Source: three-view drawing plus pictorial views. Frame: mm from the lowest corner of the part. A direction names the side the tool comes from. Round coordinates to 2 decimals unless told otherwise and drop trailing zeros. Loops run counter-clockwise (first coordinate to the right, second up) from the corner with the lowest first, then second, coordinate; pieces in that order, holes last. Notation, with made-up numbers: (65.5, 66.25) -> (84.5, 66.25) arc R27 ccw to (84.5, 100.25) -> close; hole circle Ø1 at (77, 34.5). An arc over 180 degrees is marked (long way). Put each result on its own line as item: value. Start each with the question number.
1. Contact query for flat-ended pins moving along their axis: pin 1 (2 mm diameter, centred on y = 2, z = 35.5, fed in from +X); pin 2 (2 mm diameter, centred on y = 7, z = 34.5, fed in from +X); pin 3 (2 mm diameter, centred on y = 4, z = 35, fed in from +X). Output: stop coordinate, or through.
2. Cut plane C-C (z = 34). Return the cut outline in (x, y), then the cut area to 3 significant figures.
3. Material intervals for L1, parallel to Z at x = 5, y = 5.3; L2, parallel to Z at x = 9.75, y = 3.75; L3, parallel to Z at x = 5.5, y = 3.5, sorted ascending.
4. Cut plane A-A (y = 5). Return the cut outline in (x, z), then the cut area to 3 significant figures.
5. Cut plane B-B (z = 56). Return the cut outline in (x, y).
6. Set-up query: the marked faces 1 and 2. Return all of +Z, -Z, +X, -X, +Y, -Y with unobstructed straight access to the full face (end or side cutting, diameter ignored); none if empty.
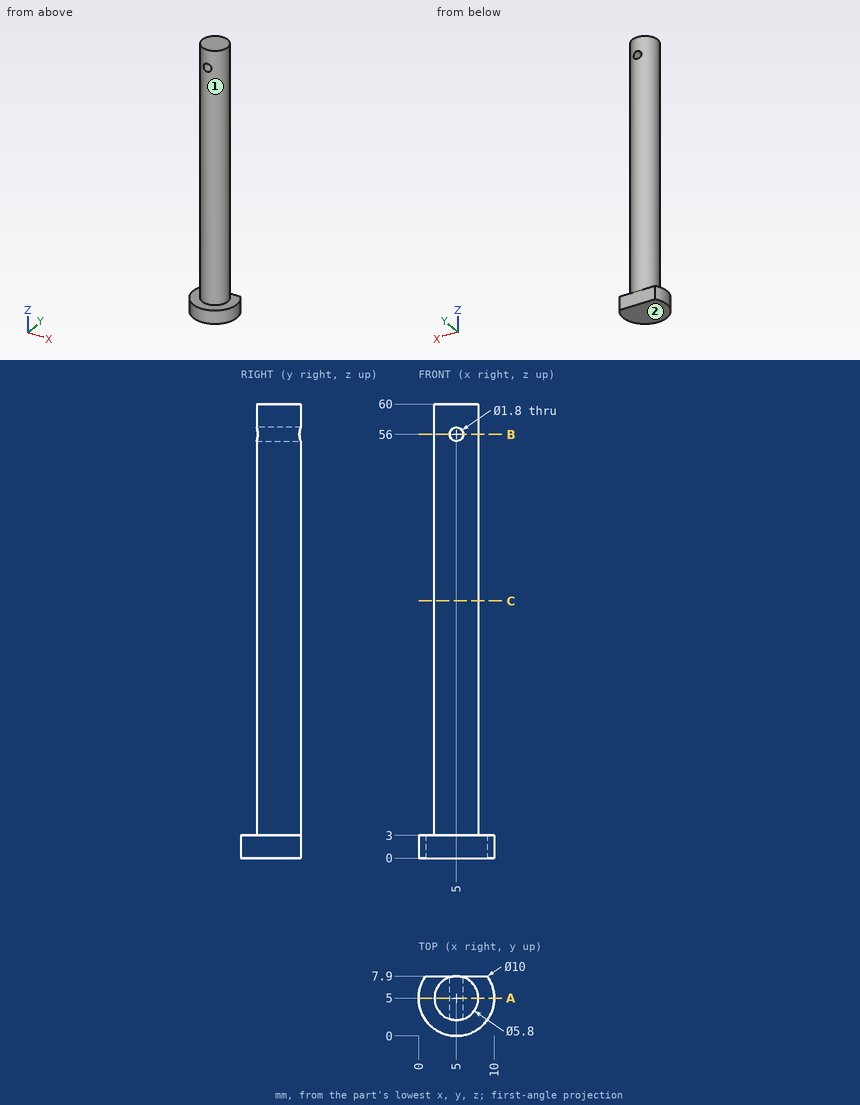
Solution:
1. pin 1: stops at x = 7.1
1. pin 2: stops at x = 7.72
1. pin 3: stops at x = 7.9
2. outline: circle Ø5.8 at (5, 5)
2. area: 26.4 mm^2
3. L1: z = 0 to 55.1, 56.9 to 60
3. L2: z = 0 to 3
3. L3: z = 0 to 55.25, 56.75 to 60
4. outline: (0, 0) -> (10, 0) -> (10, 3) -> (7.9, 3) -> (7.9, 60) -> (2.1, 60) -> (2.1, 3) -> (0, 3) -> close; hole circle Ø1.8 at (5, 56)
4. area: 358 mm^2
5. outline: (4.1, 2.24) -> (4.1, 7.76) arc R2.9 ccw to start; (5.9, 2.24) arc R2.9 ccw to (5.9, 7.76) -> close
6. face 1: +Z
6. face 2: -Z, +X, -X, +Y, -Y
